Geometry check sheet. Reference: the model listing, model coordinates, mm. Coordinates: 2 decimals unless noted, no trailing zeros. Loops run counter-clockwise (first coordinate to the right, second up) from the corner with the lowest first, then second, coordinate; pieces in that order, holes last.
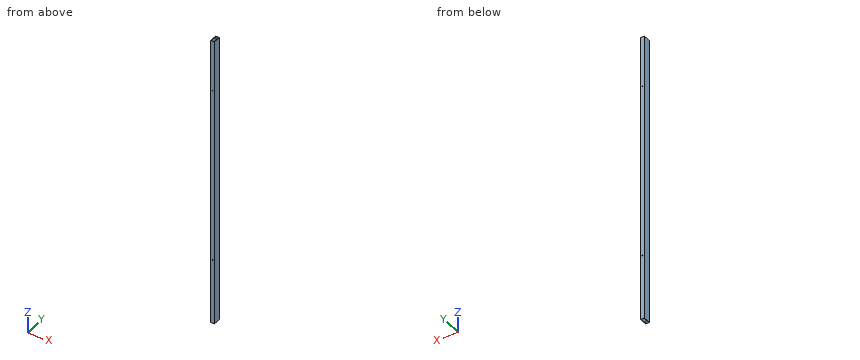
from build123d import *

# Parameters (mm, degrees)
ESQUISSE1_W                  = 25
ESQUISSE1_H                  = 50
ESQUISSE1_W_2                = 19.086637974
ESQUISSE1_H_2                = 45.621468926
BOSS_EXTRU_1_DEPTH           = 2000
ESQUISSE2_R                  = 3
ENL_V_MAT_EXTRU_1_DEPTH      = 1
ENL_V_MAT_EXTRU_1_DEPTH_BACK = 51
ESQUISSE3_R                  = 3
ENL_V_MAT_EXTRU_2_DEPTH      = 1
ENL_V_MAT_EXTRU_2_DEPTH_BACK = 51


with BuildPart() as part:
    # Esquisse1 → Boss.-Extru.1 (new body)
    with BuildSketch(Plane.XY):
        Rectangle(ESQUISSE1_W, ESQUISSE1_H)
        Rectangle(ESQUISSE1_W_2, ESQUISSE1_H_2, mode=Mode.SUBTRACT)
    extrude(amount=BOSS_EXTRU_1_DEPTH)

    # Esquisse2 → Enlèv. mat.-Extru.1 (cut, two sides)
    with BuildSketch(Plane(origin=(0, 25, 0), x_dir=(1, 0, 0), z_dir=(0, 1, 0))) as enl_v_mat_extru_1_sk:
        with Locations((0.185438708, -1648.872663575)):
            Circle(ESQUISSE2_R)
    extrude(amount=ENL_V_MAT_EXTRU_1_DEPTH, mode=Mode.SUBTRACT)
    extrude(enl_v_mat_extru_1_sk.sketch, amount=-ENL_V_MAT_EXTRU_1_DEPTH_BACK, mode=Mode.SUBTRACT)

    # Esquisse3 → Enlèv. mat.-Extru.2 (cut, two sides)
    with BuildSketch(Plane(origin=(0, 25, 0), x_dir=(1, 0, 0), z_dir=(0, 1, 0))) as enl_v_mat_extru_2_sk:
        with Locations((0.185438708, -448.872663575)):
            Circle(ESQUISSE3_R)
    extrude(amount=ENL_V_MAT_EXTRU_2_DEPTH, mode=Mode.SUBTRACT)
    extrude(enl_v_mat_extru_2_sk.sketch, amount=-ENL_V_MAT_EXTRU_2_DEPTH_BACK, mode=Mode.SUBTRACT)


solid = part.part
1) Depth check by flat-ended pin: pin 1 (8 mm diameter, centred on x = 5, y = -7, fed in from -Z). Enter the tip coordinate at first touch or a pass-through.
Data:
pin 1: passes through
2) Material ranges on probe 1 along X at (y, z) = (4, 192); probe 2 along Y at (x, z) = (-3.25, 1654), recorded low to high.
Data:
probe 1: x = -12.5 to -9.54, 9.54 to 12.5
probe 2: y = -25 to -22.81, 22.81 to 25
3) Section check B-B on z = 1551.5. Record the cut outline in (x, y).
Data:
outline: (-12.5, -25) - (12.5, -25) - (12.5, 25) - (-12.5, 25) - close; hole (-9.54, -22.81) - (9.54, -22.81) - (9.54, 22.81) - (-9.54, 22.81) - close
4) Section check A-A on y = -8.5. Record the cut outline in (x, z).
Data:
outline: (-12.5, 0) - (-9.54, 0) - (-9.54, 2000) - (-12.5, 2000) - close; (9.54, 0) - (12.5, 0) - (12.5, 2000) - (9.54, 2000) - close
